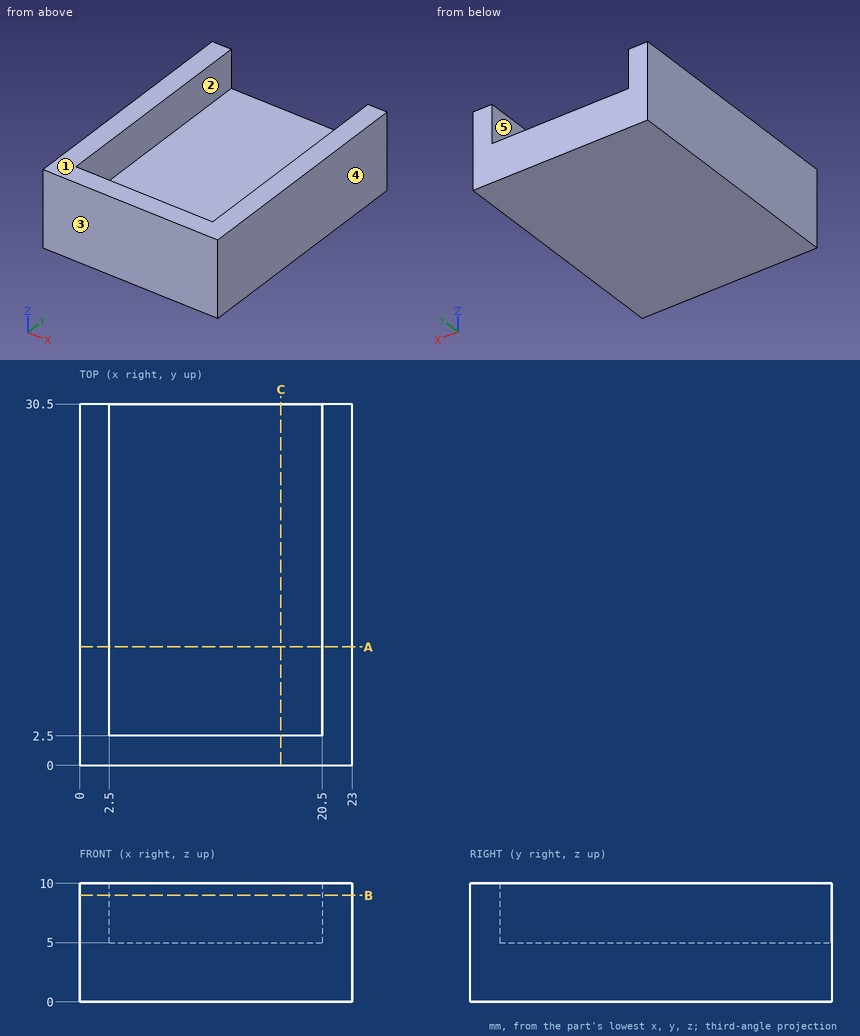
Could you check a few things on this drawing? It's one solid part, dimensions in mm from its lowest x, y, z. A direction names the side the tool comes from. Give positions to 0.01 mm unless a question says otherwise; leave off trailing zeros. Order: outer loops, then holes, each group sorted by start corner. A loop starts at its lowest first (then second) coordinate and runs counter-clockwise, first axis right, second up. Notation, with made-up numbers: (-9, -25) - (-4, -25) arc R18 cw to (-4, -2) - close; hole circle Ø11 at (79, -16). An arc over 180 degrees is marked (long way). Return JSON: item names as keys, results as strings. Group by question number.
Q1. Will these pins go through, and if not, where does the flat tip stop? pin 1 Ø12 at (x, y) = (14, 17) entering from -Z; pin 2 Ø4 at (x, y) = (10.5, 9) entering from +Z; pin 3 Ø1.5 at (x, z) = (9, 7.5) entering from +Y.
Q2. Which directions (+Z, -Z, +X, -X, +Y, -Y) give clear straight access to the entire face, cutting with the end or side of a thin tool? Please do the marked faces 1 and 2.
Q3. Please list where these lines run through material, in increasing order: line 1 along X through (y, z) = (23, 9); line 2 along Y through (x, z) = (12.75, 8.5); line 3 along Z through (x, y) = (14.25, 28.5). Write a range as [from, to].
Q4. Suppose I cut it at B-B, the plane z = 9. Please give me the cut outline in (x, y).
Q5. Thinking about a two-plate mould opening in X: for the marked faces 3, 4 and 5, which applies, pulls with the +X half, pulls with the -X half, needs draft (parallel to the pull), parting line crosses it, or undercut?
Q6. Suppose I cut it at A-A, the plane y = 10. Please give me the cut outline in (x, z), and give its area (3 significant figures).
Q7. Suppose I cut it at C-C, the plane x = 17. Please give me the cut outline in (y, z).
Resolved:
{
 "1": {"pin 1": "stops at z = 0", "pin 2": "stops at z = 5", "pin 3": "stops at y = 2.5"},
 "2": {"face 1": "+Z, +X, -X, +Y, -Y", "face 2": "+Z, +Y"},
 "3": {"line 1": "x = [0, 2.5], [20.5, 23]", "line 2": "y = [0, 2.5]", "line 3": "z = [0, 5]"},
 "4": {"outline": "(0, 0) - (23, 0) - (23, 30.5) - (20.5, 30.5) - (20.5, 2.5) - (2.5, 2.5) - (2.5, 30.5) - (0, 30.5) - close"},
 "5": {"face 3": "needs draft", "face 4": "pulls with the +X half", "face 5": "undercut"},
 "6": {"outline": "(0, 0) - (23, 0) - (23, 10) - (20.5, 10) - (20.5, 5) - (2.5, 5) - (2.5, 10) - (0, 10) - close", "area": "140 mm2"},
 "7": {"outline": "(0, 0) - (30.5, 0) - (30.5, 5) - (2.5, 5) - (2.5, 10) - (0, 10) - close"}
}
